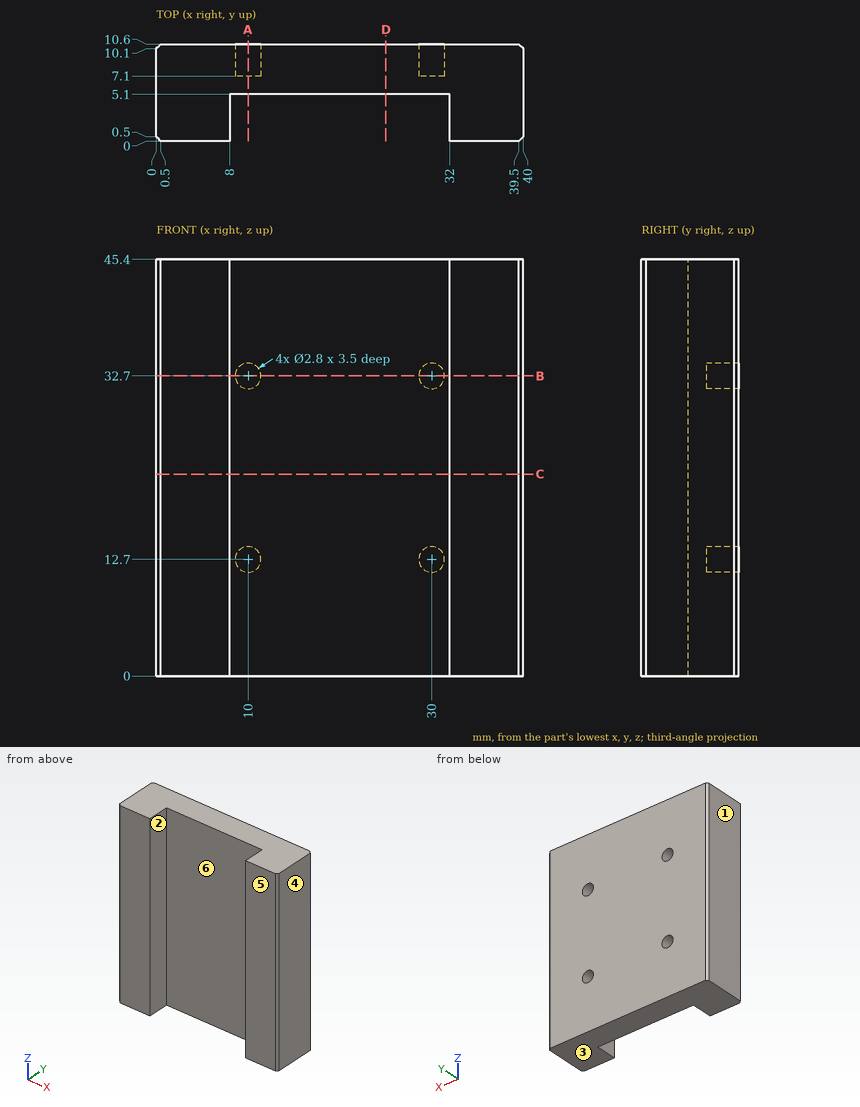
Design review of the part shown in the three views and the two pictorial views. Dimensions are in mm from the part's minimum x, y and z. A direction names the side the tool comes from. Give positions to 0.01 mm unless a question says otherwise; leave off trailing zeros. Write each loop counter-clockwise with the first axis right and the second up, starting at its lowest first coordinate (ties: lowest second). Pieces come first, ordered by that corner, then holes.
Item 1: Wall thickness on probe 1 along X at (y, z) = (9.15, 32.7); probe 2 along X at (y, z) = (3.5, 41.5); probe 3 along Y at (x, z) = (22, 25.5): over which ranges is each line inside the solid? List them lowest first.
Item 2: Take a section at C-C (z = 22). Give the boundary of the cut face in (x, y).
Item 3: Take a section at B-B (z = 32.7). Give the boundary of the cut face in (x, y), and give its area (4 significant figures).
Item 4: Take a section at A-A (x = 10). Give the boundary of the cut face in (y, z), and give its area (3 significant figures).
Item 5: Insertion check: P1, Ø2.5, axis at x = 30, z = 12.7, coming from the -Y side; P2, Ø3, axis at x = 9.5, z = 12.5, coming from the +Y side; P3, Ø1.7, axis at x = 30, z = 32.7, coming from the +Y side. Each pin has a flat end and moves straight along its axis. Give the tip position at first contact, or say it passes through.
Item 6: Machinability: for the marked faces 5 and 6, which of the approach directions +Z, -Z, +X, -X, +Y, -Y give a long, thin tool a straight path to every point of the face, cutting with its end or side? Answer none if there is none.
Item 7: The part is to be moulded in two halves that separate along X. For the marked faces 1, 2, 3 and 4, say which applies: +X half, -X half, draft (parallel to the pull), parting line (faces both ways), or undercut.
Item 8: Take a section at D-D (x = 25). Give the boundary of the cut face in (y, z).
Established:
1. probe 1: x = 0 to 8.6, 11.4 to 28.6, 31.4 to 40
1. probe 2: x = 0 to 8, 32 to 40
1. probe 3: y = 5.1 to 10.6
2. outline: (0, 0.5) - (0.5, 0) - (8, 0) - (8, 5.1) - (32, 5.1) - (32, 0) - (39.5, 0) - (40, 0.5) - (40, 10.1) - (39.5, 10.6) - (0.5, 10.6) - (0, 10.1) - close
3. outline: (0, 0.5) - (0.5, 0) - (8, 0) - (8, 5.1) - (32, 5.1) - (32, 0) - (39.5, 0) - (40, 0.5) - (40, 10.1) - (39.5, 10.6) - (31.4, 10.6) - (31.4, 7.1) - (28.6, 7.1) - (28.6, 10.6) - (11.4, 10.6) - (11.4, 7.1) - (8.6, 7.1) - (8.6, 10.6) - (0.5, 10.6) - (0, 10.1) - close
3. area: 281.5 mm2
4. outline: (5.1, 0) - (10.6, 0) - (10.6, 11.3) - (7.1, 11.3) - (7.1, 14.1) - (10.6, 14.1) - (10.6, 31.3) - (7.1, 31.3) - (7.1, 34.1) - (10.6, 34.1) - (10.6, 45.4) - (5.1, 45.4) - close
4. area: 230 mm2
5. P1: stops at y = 5.1
5. P2: stops at y = 10.6
5. P3: stops at y = 7.1
6. face 5: +Z, -Z, +X, -X, -Y
6. face 6: +Z, -Z, -Y
7. face 1: -X half
7. face 2: undercut
7. face 3: draft
7. face 4: +X half
8. outline: (5.1, 0) - (10.6, 0) - (10.6, 45.4) - (5.1, 45.4) - close
